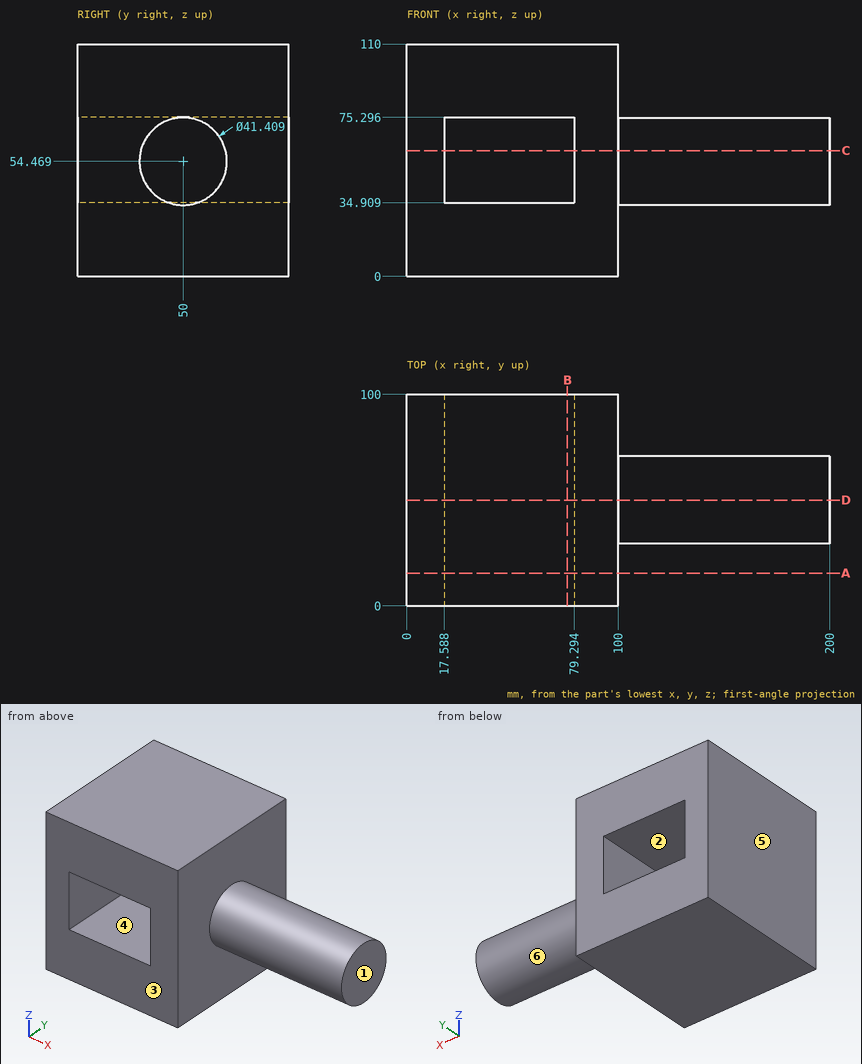
Print and shaded views of the part. All mm, measured from the part's lowest x, y and z. A direction names the side the tool comes from. Round coordinates to 2 decimals unless told otherwise and drop trailing zeros. Order: outer loops, then holes, each group sorted by start corner. A loop starts at its lowest first (then second) coordinate and runs counter-clockwise, first axis right, second up.
Q1. Slice it at D-D (y = 50). Write the cut outline in (x, z) (1 decimal).
Q2. Drop flat-ended pins along their axis: pin 1 (6 mm diameter, centred on y = 34.5, z = 94, fed in from -X); pin 2 (5 mm diameter, centred on x = 146.5, y = 66, fed in from +Z); pin 3 (10 mm diameter, centred on x = 152, y = 38.5, fed in from -Z); pin 4 (5 mm diameter, centred on x = 105, z = 51.5, fed in from -Y). Give the stop position or say it passes through.
Q3. Wall check: L1, parallel to X at y = 13, z = 66.5 (1 decimal); L2, parallel to Z at x = 57, y = 42 (1 decimal); L3, parallel to Z at x = 122, y = 49. Give the ranges that are in metal, low to high.
Q4. Which spindle directions (+Z, -Z, +X, -X, +Y, -Y) get a long thin tool onto all of the face, cutting with end or side? Do the marked faces 4, 5 and 6. Say none if no direction does.
Q5. Slice it at B-B (x = 76). Write the cut outline in (y, z) (1 decimal).
Q6. Slice it at A-A (y = 15.5). Write the cut outline in (x, z) (1 decimal), and give its area (3 significant figures).
Q7. Two-plate mould, pull along X, no slides. Class the marked faces 1, 2 and 3: pulls with the +X half, pulls with the -X half, needs draft (parallel to the pull), parting line crosses it, or undercut.
Q8. Slice it at C-C (z = 59.5). Write the cut outline in (x, y) (1 decimal), and give its area (3 significant figures).
Results below:
1. outline: (0, 0) - (100, 0) - (100, 33.8) - (200, 33.8) - (200, 75.2) - (100, 75.2) - (100, 110) - (0, 110) - close; hole (17.6, 34.9) - (79.3, 34.9) - (79.3, 75.3) - (17.6, 75.3) - close
2. pin 1: stops at x = 0
2. pin 2: stops at z = 70.17
2. pin 3: stops at z = 34.81
2. pin 4: stops at y = 29.3
3. L1: x = 0 to 17.6, 79.3 to 100
3. L2: z = 0 to 34.9, 75.3 to 110
3. L3: z = 33.79 to 75.15
4. face 4: +Y, -Y
4. face 5: +Z, -Z, -X, +Y, -Y
4. face 6: +X
5. outline: (0, 0) - (100, 0) - (100, 34.9) - (0, 34.9) - close; (0, 75.3) - (100, 75.3) - (100, 110) - (0, 110) - close
6. outline: (0, 0) - (100, 0) - (100, 110) - (0, 110) - close; hole (17.6, 34.9) - (79.3, 34.9) - (79.3, 75.3) - (17.6, 75.3) - close
6. area: 8,510 mm2
7. face 1: pulls with the +X half
7. face 2: undercut
7. face 3: needs draft
8. outline: (0, 0) - (17.6, 0) - (17.6, 100) - (0, 100) - close; (79.3, 0) - (100, 0) - (100, 29.9) - (200, 29.9) - (200, 70.1) - (100, 70.1) - (100, 100) - (79.3, 100) - close
8. area: 7,850 mm2
